The listing builds one solid part. Answer for the finished solid, in the listing's coordinates (mm). Face numbers are marked on the shaded views. A direction names the side the tool comes from. Round coordinates to 2 decimals unless told otherwise and drop trailing zeros. Loops run counter-clockwise (first coordinate to the right, second up) from the corner with the lowest first, then second, coordinate; pieces in that order, holes last. Notation, with made-up numbers: (39, 0.5) -> (73, 0.5) arc R29 ccw to (73, 35.5) -> close; hole circle Ø3 at (68, 8.5). An arc over 180 degrees is marked (long way). Use a Markdown table: item, result. Add a question column.
Q1. Section C-C on z = -4.75 is taken. Give the vertices of the cut face in (x, y) (3 decimals), then the cut area to 3 significant figures.
Q2. Which of the six approach directions +Z, -Z, +X, -X, +Y, -Y give full straight-line access (tool end or side, diameter ignored) to the marked faces 1, 2, 3 and 4?
Q3. Section B-B on y = 40 is taken. Give the vertices of the cut face in (x, z).
Q4. Given pin 1 Ø4.5 at (y, z) = (46, -9) entering from +X; pin 2 Ø4 at (y, z) = (2.5, -7.5) entering from -X; pin 3 Ø1.4 at (x, z) = (-19, -6.5) entering from +Y, each flat-ended and moving along its own axis, determine where each tip first touches the part or whether it passes through.
Q5. Section D-D on y = 15.5 is taken. Give the vertices of the cut face in (x, z), then the cut area to 3 significant figures.
Q6. Section A-A on x = -8.5 is taken. Give the vertices of the cut face in (y, z).
Q7. Consider line 1 (Y direction, x = -2, z = -11); line 2 (Y direction, x = -26, z = -10.5); line 3 (X direction, y = 41.5, z = -14). Determine where each line is inside the solid, lowest interval first.
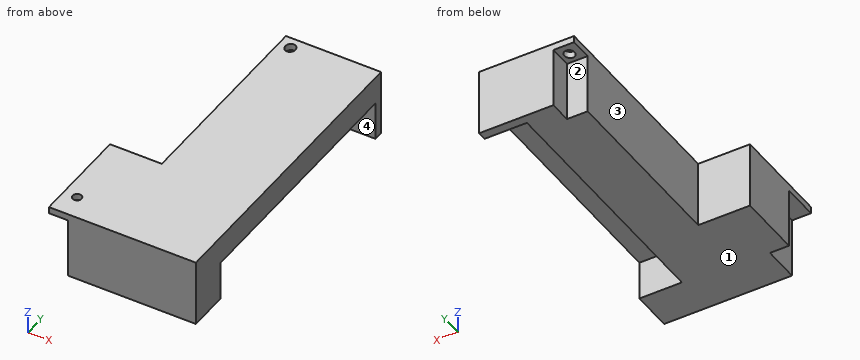
from build123d import *

# Parameters (mm, degrees)
F0_R     = 1.016
F1_DEPTH = 15.24
F2_W     = 4.318
F2_H     = 8.255
F2_R     = 1.016
F3_DEPTH = 13.716
F4_W     = 4.699
F4_H     = 5.08
F5_DEPTH = 13.716
F6_W     = 58.039
F6_H     = 8.89
F7_DEPTH = 9.652


with BuildPart() as f1:
    # F0 (on Top) → F1 (new body)
    with BuildSketch(Plane.XY):
        Polygon((0, 69.342), (-21.59, 69.342), (-21.59, 22.86), (-33.3502, 22.86), (-33.3502, 9.144), (0, 9.144), align=None)
        with BuildLine():
            add(Edge.make_bspline(
                [(-18.923, 67.9196), (-20.902734, 67.9196), (-19.912867, 65.9765), (-18.923, 64.0334), (-17.933133, 65.9765), (-16.943266, 67.9196), (-18.923, 67.9196)],
                knots=[0, 0, 0, 2.094395, 2.094395, 4.18879, 4.18879, 6.283185, 6.283185, 6.283185], degree=2, weights=[1, 0.5, 1, 0.5, 1, 0.5, 1]))
        make_face(mode=Mode.SUBTRACT)
        Polygon((0, 0), (0, 9.144), (-33.3502, 9.144), (-33.3502, 0), (-21.59, 0), align=None)
        with Locations((-30.2768, 5.461)):
            Circle(F0_R, mode=Mode.SUBTRACT)
    extrude(amount=-F1_DEPTH)

    # F2 (on face) → F3 (cut)
    with BuildSketch(Plane(origin=(0, 0, -15.24), x_dir=(1, 0, 0), z_dir=(0, 0, -1))):
        with Locations((-31.1912, -4.1275)):
            Rectangle(F2_W, F2_H)
        with Locations((-30.2768, -5.461)):
            Circle(F2_R, mode=Mode.SUBTRACT)
    extrude(amount=-F3_DEPTH, mode=Mode.SUBTRACT)

    # F4 (on face) → F5 (cut)
    with BuildSketch(Plane(origin=(0, 0, -15.24), x_dir=(1, 0, 0), z_dir=(0, 0, -1))):
        with Locations((-19.2405, -66.802)):
            Rectangle(F4_W, F4_H)
    extrude(amount=-F5_DEPTH, mode=Mode.SUBTRACT)

    # F6 (on face) → F7 (cut)
    with BuildSketch(Plane.YZ):
        with Locations((38.2905, -10.795)):
            Rectangle(F6_W, F6_H)
    extrude(amount=-F7_DEPTH, mode=Mode.SUBTRACT)


solid = f1.part
Checked values:
| question | item | result |
|---|---|---|
| 1 | outline | (-33.35, 8.255) -> (-29.032, 8.255) -> (-29.032, 0) -> (0, 0) -> (0, 69.342) -> (-16.891, 69.342) -> (-16.891, 64.262) -> (-21.59, 64.262) -> (-21.59, 22.86) -> (-33.35, 22.86) -> close |
| 1 | area | 1,710 mm2 |
| 2 | face 1 | -Z, +X, -X, +Y, -Y |
| 2 | face 2 | -Z, -X, +Y |
| 2 | face 3 | +Z, -Z, -X, +Y |
| 2 | face 4 | -Z, +X |
| 3 | outline | (-21.59, -15.24) -> (-9.65, -15.24) -> (-9.65, -6.35) -> (0, -6.35) -> (0, 0) -> (-21.59, 0) -> close |
| 4 | pin 1 | stops at x = -9.65 |
| 4 | pin 2 | stops at x = -29.03 |
| 4 | pin 3 | stops at y = 64.26 |
| 5 | outline | (-33.35, -15.24) -> (-9.65, -15.24) -> (-9.65, -6.35) -> (0, -6.35) -> (0, 0) -> (-33.35, 0) -> close |
| 5 | area | 422 mm2 |
| 6 | outline | (0, -15.24) -> (9.27, -15.24) -> (9.27, -6.35) -> (67.31, -6.35) -> (67.31, -15.24) -> (69.34, -15.24) -> (69.34, 0) -> (0, 0) -> close |
| 7 | line 1 | y = 0 to 9.27, 67.31 to 69.34 |
| 7 | line 2 | y = 0 to 22.86 |
| 7 | line 3 | x = -21.59 to -9.65 |
